from build123d import *

# Parameters (mm, degrees)
PRISM001_DEPTH            = 14
PRISM001_ROLL_ANGLE       = 90.000052
PRISM001_PITCH_ANGLE      = 59.999967
PRISM001_PLACEMENT_ANGLE  = 90.000052
CYLINDER_R                = 2
CYLINDER_DEPTH            = 20
CYLINDER_PITCH_ANGLE      = 90
FUSION002_PLACEMENT_ANGLE = -90
FUSION003_PLACEMENT_ANGLE = -90
BOX_W                     = 36
BOX_H                     = 38
BOX_DEPTH                 = 8
PAD_DEPTH                 = 20
CHAMFER_SIZE              = 3
FILLET_R                  = 26


with BuildPart() as prism001:
    # Prism001 → Prism001 (new body)
    with BuildSketch(Plane.XY):
        Polygon((4, 0), (2, 3.464102), (-2, 3.464102), (-4, 0), (-2, -3.464102), (2, -3.464102), align=None)
    extrude(amount=PRISM001_DEPTH)


with BuildPart() as prism001_1:
    # Prism001 roll: moved
    add(prism001.part.rotate(Axis((0, 0, 0), (1, 0, 0)), PRISM001_ROLL_ANGLE))


with BuildPart() as prism001_2:
    # Prism001 pitch: moved
    add(prism001_1.part.rotate(Axis((0, 0, 0), (0, 1, 0)), PRISM001_PITCH_ANGLE))


with BuildPart() as prism001_3:
    # Prism001 placement: moved
    add(prism001_2.part.moved(Location((5, 9, 10))).rotate(Axis((5, 9, 10), (0, 0, 1)), PRISM001_PLACEMENT_ANGLE))


with BuildPart() as cylinder:
    # Cylinder → Cylinder (new body)
    with BuildSketch(Plane.XY):
        Circle(CYLINDER_R)
    extrude(amount=CYLINDER_DEPTH)


with BuildPart() as cylinder_1:
    # Cylinder pitch: moved
    add(cylinder.part.rotate(Axis((0, 0, 0), (0, 1, 0)), CYLINDER_PITCH_ANGLE))


with BuildPart() as cylinder_2:
    # Cylinder placement: moved
    add(cylinder_1.part.moved(Location((-3, 9, 10))))


with BuildPart() as fusion002:
    # Fusion002 base: copy of Cylinder
    add(cylinder_2.part)

    # Fusion002: union Prism001
    add(prism001_3.part)


with BuildPart() as fusion002_1:
    # Fusion002 placement: moved
    add(fusion002.part.moved(Location((14, 50, 0))).rotate(Axis((14, 50, 0), (0, 0, 1)), FUSION002_PLACEMENT_ANGLE))


with BuildPart() as fusion:
    # Fusion base: copy of Cylinder
    add(cylinder_2.part)

    # Fusion: union Prism001
    add(prism001_3.part)


with BuildPart() as fusion_1:
    # Fusion placement: moved
    add(fusion.part.moved(Location((0, 18, 0))))


with BuildPart() as fusion001:
    # Fusion001 base: copy of Cylinder
    add(cylinder_2.part)

    # Fusion001: union Prism001
    add(prism001_3.part)


with BuildPart() as fusion004:
    # Fusion003 base: copy of Cylinder
    add(cylinder_2.part)

    # Fusion003: union Prism001
    add(prism001_3.part)


with BuildPart() as fusion004_1:
    # Fusion003 placement: moved
    add(fusion004.part.moved(Location((32, 50, 0))).rotate(Axis((32, 50, 0), (0, 0, 1)), FUSION003_PLACEMENT_ANGLE))

    # Fusion004: union Fusion002, Fusion, Fusion001
    add(fusion002_1.part)
    add(fusion_1.part)
    add(fusion001.part)


with BuildPart() as cube:
    # Box → Box (new body)
    with BuildSketch(Plane(origin=(8, 4, 6), x_dir=(1, 0, 0), z_dir=(0, 0, 1))):
        with Locations((18, 19)):
            Rectangle(BOX_W, BOX_H)
    extrude(amount=BOX_DEPTH)


with BuildPart() as cut001:
    # Sketch → Pad (new body)
    with BuildSketch(Plane.XY):
        Polygon((0, 0), (8, 0), (8, 42), (50, 42), (50, 50), (0, 50), align=None)
    extrude(amount=PAD_DEPTH)

    # Chamfer
    chamfer_edges = [cut001.edges().sort_by_distance(p)[0] for p in [
        (4, 0, 0),
        (4, 0, 20),
        (50, 46, 0),
        (50, 46, 20),
        (0, 50, 10),
    ]]
    chamfer(chamfer_edges, length=CHAMFER_SIZE)

    # Fillet
    fillet_edges = [cut001.edges().sort_by_distance(p)[0] for p in [
        (8, 42, 10),
    ]]
    fillet(fillet_edges, radius=FILLET_R)

    # Cut: cut Cube
    add(cube.part, mode=Mode.SUBTRACT)

    # Cut001: cut Fusion004
    add(fusion004_1.part, mode=Mode.SUBTRACT)


solid = cut001.part
For this review, take the finished solid that the model builds, in its own axes (mm). A direction names the side the tool comes from. Round coordinates to 2 decimals unless told otherwise and drop trailing zeros. Write each loop counter-clockwise with the first axis right and the second up, starting at its lowest first coordinate (ties: lowest second). Pieces come first, ordered by that corner, then holes. Notation, with made-up numbers: (67, -36) - (98, -36) arc R22 ccw to (98, -5) - close; hole circle Ø11 at (-11.5, 49). An arc over 180 degrees is marked (long way). Use a Markdown table: item, result.
Q1. We need section A-A (y = 27). Give the boundary of the cut face in (x, z), plus the area to 3 significant figures.
Derived:
| item | result |
|---|---|
| outline | (0, 0) - (10.44, 0) - (10.44, 6) - (8, 6) - (8, 6.54) - (5, 6.54) - (5, 8) - (0, 8) - close; (0, 12) - (5, 12) - (5, 13.46) - (8, 13.46) - (8, 14) - (10.44, 14) - (10.44, 20) - (0, 20) - close |
| area | 149 mm2 |
Q2. Wall thickness on line 1 along X through (y, z) = (46.3, 10); line 2 along Z through (x, y) = (12.5, 41); line 3 along X through (y, z) = (48.1, 10): over which ranges is each line inside the solid? List them lowest first.
Derived:
| item | result |
|---|---|
| line 1 | x = 0 to 21, 25 to 39, 43 to 50 |
| line 2 | z = 0 to 6, 14 to 20 |
| line 3 | x = 1.1 to 21, 25 to 39, 43 to 50 |
Q3. We need section C-C (z = 4.5). Give the boundary of the cut face in (x, y).
Derived:
| item | result |
|---|---|
| outline | (0, 0) - (8, 0) - (8, 16) arc R26 cw to (34, 42) - (50, 42) - (50, 50) - (3, 50) - (0, 47) - close |
Q4. We need section B-B (x = 23). Give the boundary of the cut face in (y, z), plus the area to 3 significant figures.
Derived:
| item | result |
|---|---|
| outline | (39.56, 0) - (50, 0) - (50, 8) - (45, 8) - (45, 6.54) - (42, 6.54) - (42, 6) - (39.56, 6) - close; (39.56, 14) - (42, 14) - (42, 13.46) - (45, 13.46) - (45, 12) - (50, 12) - (50, 20) - (39.56, 20) - close |
| area | 149 mm2 |
Q5. We need section D-D (y = 41). Give the boundary of the cut face in (x, z).
Derived:
| item | result |
|---|---|
| outline | (0, 0) - (26.86, 0) - (26.86, 6) - (8, 6) - (8, 14) - (26.86, 14) - (26.86, 20) - (0, 20) - close |
Q6. Clearance check with flat-ended pins moving along their axes: pin 1 (5.5 mm diameter, centred on x = 42.5, z = 10.5, fed in from -Y); pin 2 (5.5 mm diameter, centred on y = 9, z = 11.5, fed in from +X); pin 3 (3 mm diameter, centred on y = 38.5, z = 6.5, fed in from +X). State where each tip first meets the part, or that it passes through.
Derived:
| item | result |
|---|---|
| pin 1 | stops at y = 42 |
| pin 2 | stops at x = 8 |
| pin 3 | stops at x = 23.8 |
Q7. The part is to be moulded in two halves that separate along Z. For faces 5 (the flat face through (27, 50, 10)), 6 (the flat face through (13, 37, 0)), 7 (the flat face through (37.986, 43.521, 8.292)), say which applies: pulls with the +Z half, pulls with the -Z half, needs draft (parallel to the pull), parting line crosses it, or undercut.
Derived:
| item | result |
|---|---|
| face 5 | needs draft |
| face 6 | pulls with the -Z half |
| face 7 | undercut |
Q8. Machinability: for faces 1 (the flat face through (6.479, 5.986, 8.292)), 2 (the flat face through (44.014, 43.521, 11.708)), 3 (the flat face through (13, 36, 6)), 4 (the flat face through (50, 46, 10)), which of the approach directions +Z, -Z, +X, -X, +Y, -Y give a long, thin tool a straight path to every point of the face, cutting with its end or side? Answer none if there is none.
Derived:
| item | result |
|---|---|
| face 1 | +X |
| face 2 | -Y |
| face 3 | +X, -Y |
| face 4 | +Z, -Z, +X, +Y, -Y |
